```python
from build123d import *

# Parameters (mm, degrees)
RESSALTO_EXTRUS_O1_DEPTH = 8
ESBO_O2_W                = 59
ESBO_O2_H                = 85
ESBO_O2_W_2              = 55
ESBO_O2_H_2              = 81
RESSALTO_EXTRUS_O2_DEPTH = 5
ESBO_O3_R                = 1
CORTE_EXTRUS_O1_DEPTH    = 161.48856651
ESBO_O5_W                = 74
ESBO_O5_H                = 24
ESBO_O5_W_2              = 70
ESBO_O5_H_2              = 20
RESSALTO_EXTRUS_O4_DEPTH = 5
ESBO_O6_W                = 2
ESBO_O6_H                = 19
CORTE_EXTRUS_O2_DEPTH    = 4
ESBO_O7_R                = 1
ESBO_O7_W                = 7
ESBO_O7_H                = 15
CORTE_EXTRUS_O4_DEPTH    = 161.490657476


with BuildPart() as part:
    # Esboço1 → Ressalto-extrusão1 (new body)
    with BuildSketch(Plane.XY):
        Polygon((39.408169461, 102.513026677), (39.408169461, 62.513026677), (21.778007881, 62.513026677), (21.778007881, 2.513026677), (66.778007881, 2.513026677), (66.778007881, -17.486973323), (-123.221992119, -17.486973323), (-123.221992119, 2.513026677), (-78.221992119, 2.513026677), (-78.221992119, 62.513026677), (-100.591830539, 62.513026677), (-100.591830539, 102.513026677), align=None)
    extrude(amount=RESSALTO_EXTRUS_O1_DEPTH)

    # Esboço2 → Ressalto-extrusão2 (add)
    with BuildSketch(Plane.XY.offset(8)):
        with Locations((-28.221992119, 33.013026677)):
            Rectangle(ESBO_O2_W, ESBO_O2_H)
        with Locations((-28.221992119, 33.013026677)):
            Rectangle(ESBO_O2_W_2, ESBO_O2_H_2, mode=Mode.SUBTRACT)
    extrude(amount=RESSALTO_EXTRUS_O2_DEPTH)

    # Esboço3 → Corte-extrusão1 (cut, through all)
    with BuildSketch(Plane.XY.offset(8)):
        with Locations((-13.221992119, -15.486973323)):
            Circle(ESBO_O3_R)
        with Locations((-43.099997489, -15.486973323)):
            Circle(ESBO_O3_R)
    extrude(amount=-CORTE_EXTRUS_O1_DEPTH, mode=Mode.SUBTRACT)

    # Esboço5 → Ressalto-extrusão4 (add)
    with BuildSketch(Plane.XY.offset(8)):
        with Locations((-30.591830539, 90.516300144)):
            Rectangle(ESBO_O5_W, ESBO_O5_H)
        with Locations((-30.591830539, 90.516300144)):
            Rectangle(ESBO_O5_W_2, ESBO_O5_H_2, mode=Mode.SUBTRACT)
    extrude(amount=RESSALTO_EXTRUS_O4_DEPTH)

    # Esboço6 → Corte-extrusão2 (cut)
    with BuildSketch(Plane.XY.offset(13)):
        with Locations((5.408169461, 90.516300144)):
            Rectangle(ESBO_O6_W, ESBO_O6_H)
    extrude(amount=-CORTE_EXTRUS_O2_DEPTH, mode=Mode.SUBTRACT)

    # Esboço7 → Corte-extrusão4 (cut, through all)
    with BuildSketch(Plane.XY.offset(8)):
        with Locations((-70.971992119, 55.851364498)):
            Circle(ESBO_O7_R)
        with Locations((14.528007881, 37.851364498)):
            Circle(ESBO_O7_R)
        with Locations((7.028007881, 46.851364498)):
            Rectangle(ESBO_O7_W, ESBO_O7_H)
        with Locations((14.528007881, 55.851364498)):
            Circle(ESBO_O7_R)
        with Locations((-63.471992119, 46.851364498)):
            Rectangle(ESBO_O7_W, ESBO_O7_H)
        with Locations((-70.971992119, 37.851364498)):
            Circle(ESBO_O7_R)
    extrude(amount=-CORTE_EXTRUS_O4_DEPTH, mode=Mode.SUBTRACT)


solid = part.part
```
The model under review builds one solid part; all positions refer to its coordinate system, in mm. A direction names the side the tool comes from. Round coordinates to 2 decimals unless told otherwise and drop trailing zeros. Write each loop counter-clockwise with the first axis right and the second up, starting at its lowest first coordinate (ties: lowest second). Pieces come first, ordered by that corner, then holes. Notation, with made-up numbers: M 20.25,13 L 49.25,13 A17 ccw 49.25,21 Z; hole C 82,22 d4. An arc over 180 degrees is marked long. Use CSV: the item, a comma, the result in double quotes. Start each with the question number.
(1) We need section B-B, the plane x = 34. State the section outline as (y, z) points.
(2) We need section A-A, the plane y = 42.5. State the section outline as (x, z) points.
(3) The part is to be moulded in two halves that separate along X. For faces 1 (the face through (6.408, 90.3, 8.8)), 2 (the face through (-31, 102.516, 10)), 3 (the face through (-29, 73.513, 10)), say which applies: +X half, -X half, draft (parallel to the pull), parting line (faces both ways), or undercut.
(4) For line 1 along Y through (x, z) = (-3, 12.25); line 2 along X through (y, z) = (44, 3); line 3 along Y through (x, z) = (-57, 9), list the stretches that pass through material, from the lowest coordinate up.
(5) We need section C-C, the plane z = 4.25. State how many separate pieces and enclosed holes the cut face has, then the cut area to 3 significant figures.
(6) Tool access review of faces 4 (the face through (-100.592, 82, 4)), 5 (the face through (7, 54.351, 4)), 6 (the face through (1.278, 32, 10)), 7 (the face through (-67.592, 90, 10)): name each direction out of +Z, -Z, +X, -X, +Y, -Y from which nothing blocks a thin tool from reaching the whole face with its end or side.
(7) Clearance check with flat-ended pins moving along their axes: P1, Ø6.5, axis at y = 42.5, z = 2, coming from the -X side; P2, Ø3, axis at x = -70.97, y = 37.85, coming from the +Z side; P3, Ø1.6, axis at x = 5, z = 10.5, coming from the -Y side. State where each tip first meets the part, or that it passes through.
(8) We need section D-D, the plane y = -5. State the section outline as (x, z) points, then the cut area to 3 significant figures.
Findings:
1,outline,"M -17.49,0 L 2.51,0 L 2.51,8 L -17.49,8 Z; M 62.51,0 L 102.51,0 L 102.51,8 L 62.51,8 Z"
2,outline,"M -78.22,0 L -66.97,0 L -66.97,8 L -78.22,8 Z; M -59.97,0 L 3.53,0 L 3.53,8 L 1.28,8 L 1.28,13 L -0.72,13 L -0.72,8 L -55.72,8 L -55.72,13 L -57.72,13 L -57.72,8 L -59.97,8 Z; M 10.53,0 L 21.78,0 L 21.78,8 L 10.53,8 Z"
3,face 1,"+X half"
3,face 2,"draft"
3,face 3,"undercut"
4,line 1,"-9.49 to -7.49, 73.51 to 75.51, 78.52 to 80.52, 100.52 to 102.52"
4,line 2,"-78.22 to -66.97, -59.97 to 3.53, 10.53 to 21.78"
4,line 3,"-9.49 to 75.51, 78.52 to 80.52, 100.52 to 102.52"
5,separate pieces,"1"
5,enclosed holes,"8"
5,area,"15,200 mm^2"
6,face 4,"+Z, -Z, -X, +Y"
6,face 5,"+Z, -Z"
6,face 6,"+Z, +X, -Y"
6,face 7,"+Z, -X, +Y, -Y"
7,P1,"x = -78.22"
7,P2,"z = 8"
7,P3,"y = 78.52"
8,outline,"M -123.22,0 L 66.78,0 L 66.78,8 L 1.28,8 L 1.28,13 L -0.72,13 L -0.72,8 L -55.72,8 L -55.72,13 L -57.72,13 L -57.72,8 L -123.22,8 Z"
8,area,"1,540 mm^2"
